```python
from build123d import *

# Parameters (mm, degrees)
SKETCH1_W           = 50
SKETCH1_H           = 32
BOSS_EXTRUDE1_DEPTH = 13
SKETCH2_W           = 15
SKETCH2_H           = 22
BOSS_EXTRUDE2_DEPTH = 13
SKETCH3_W           = 6.961388266
SKETCH3_H           = 22
BOSS_EXTRUDE3_DEPTH = 32
SKETCH4_W           = 19
SKETCH4_H           = 12
BOSS_EXTRUDE4_DEPTH = 15
BOSS_EXTRUDE5_DEPTH = 15


with BuildPart() as part:
    # Sketch1 → Boss-Extrude1 (new body)
    with BuildSketch(Plane(origin=(0, 0, 0), x_dir=(1, 0, 0), z_dir=(0, 1, 0))):
        Rectangle(SKETCH1_W, SKETCH1_H)
    extrude(amount=BOSS_EXTRUDE1_DEPTH)

    # Sketch2 → Boss-Extrude2 (add)
    with BuildSketch(Plane(origin=(0, 0, -16), x_dir=(-1, 0, 0), z_dir=(0, 0, -1))):
        with Locations((17.5, 24)):
            Rectangle(SKETCH2_W, SKETCH2_H)
    extrude(amount=-BOSS_EXTRUDE2_DEPTH)

    # Sketch3 → Boss-Extrude3 (add)
    with BuildSketch(Plane.XY.offset(16)):
        with Locations((-6.519305867, 24)):
            Rectangle(SKETCH3_W, SKETCH3_H)
    extrude(amount=-BOSS_EXTRUDE3_DEPTH)

    # Sketch4 → Boss-Extrude4 (add)
    with BuildSketch(Plane(origin=(0, 0, -16), x_dir=(-1, 0, 0), z_dir=(0, 0, -1))):
        with Locations((-6.461388266, 19)):
            Rectangle(SKETCH4_W, SKETCH4_H)
    extrude(amount=-BOSS_EXTRUDE4_DEPTH)

    # Sketch5 → Boss-Extrude5 (add)
    with BuildSketch(Plane(origin=(0, 0, -16), x_dir=(-1, 0, 0), z_dir=(0, 0, -1))):
        Polygon((-15.961388266, 25), (3.038611734, 35), (3.038611734, 25), align=None)
    extrude(amount=-BOSS_EXTRUDE5_DEPTH)


solid = part.part
```
The model under review builds one solid part; all positions refer to its coordinate system, in mm. A direction names the side the tool comes from. Give positions to 0.01 mm unless a question says otherwise; leave off trailing zeros. Loops run counter-clockwise (first coordinate to the right, second up) from the corner with the lowest first, then second, coordinate; pieces in that order, holes last. Notation, with made-up numbers: (58, 44) -> (67, 44) arc R38 ccw to (67, 83) -> close; hole circle Ø2 at (-3, -12.5). An arc over 180 degrees is marked (long way). Use CSV: the item, a comma, the result in double quotes.
1. Consider section A-A, the plane z = -4. Write out the cut boundary in (x, y).
Result:
outline,"(-25, 0) -> (25, 0) -> (25, 13) -> (15.96, 13) -> (15.96, 25) -> (-3.04, 35) -> (-25, 35) -> close"
2. For P1, Ø5.5, axis at y = 25, z = 11, coming from the -X side; P2, Ø4.5, axis at x = -16, z = 10, coming from the +Y side; P3, Ø8, axis at y = 31, z = 9.5, coming from the +X side, all flat-tipped, find the tip position at first contact; note any pin that passes through.
Result:
P1,"stops at x = -10"
P2,"stops at y = 13"
P3,"stops at x = -3.04"
3. Consider section D-D, the plane z = 6.5. Write out the cut boundary in (x, y).
Result:
outline,"(-25, 0) -> (25, 0) -> (25, 13) -> (-3.04, 13) -> (-3.04, 35) -> (-10, 35) -> (-10, 13) -> (-25, 13) -> close"
4. To check wall thickness, follow probe 1 along Z at (x, y) = (-1, 15); probe 2 along Y at (x, z) = (5, 9.5); probe 3 along X at (y, z) = (19, 6). State the ranges of each line that lie inside material, in increasing order. Write a range as from..to.
Result:
probe 1,"z = -16..-1"
probe 2,"y = 0..13"
probe 3,"x = -10..-3.04"
5. Consider section C-C, the plane x = -18. Write out the cut boundary in (y, z), then the cut area to 3 significant figures.
Result:
outline,"(0, -16) -> (35, -16) -> (35, -3) -> (13, -3) -> (13, 16) -> (0, 16) -> close"
area,"702 mm²"
6. Consider section B-B, the plane y = 16.5. Write out the cut boundary in (x, z).
Result:
outline,"(-25, -16) -> (15.96, -16) -> (15.96, -1) -> (-3.04, -1) -> (-3.04, 16) -> (-10, 16) -> (-10, -3) -> (-25, -3) -> close"
7. Machinability: for faces 1 (the face through (-17, 24, -3)), 2 (the face through (0, 0, 0)), 3 (the face through (-3.039, 24, 8)), 4 (the face through (15.961, 19, -9)), which of the approach directions +Z, -Z, +X, -X, +Y, -Y give a long, thin tool a straight path to every point of the face, cutting with its end or side? Answer none if there is none.
Result:
face 1,"+Z, -X, +Y"
face 2,"+Z, -Z, +X, -X, -Y"
face 3,"+Z, +X, +Y"
face 4,"+Z, -Z, +X, +Y"
